Input: part model. Units: mm. Frame: model coordinates. A direction names the side the tool comes from. Round coordinates to 2 decimals unless told otherwise and drop trailing zeros. Answer as a JSON object with one key per item and string values.
```python
from build123d import *

# Parameters (mm, degrees)
SKETCH2_R           = 9.25
BOSS_EXTRUDE1_DEPTH = 4
SKETCH3_R           = 4.5
BOSS_EXTRUDE2_DEPTH = 1.2


with BuildPart() as part:
    # Sketch2 → Boss-Extrude1 (new, symmetric)
    with BuildSketch(Plane(origin=(0, 0, 0), x_dir=(1, 0, 0), z_dir=(0, 1, 0))):
        with BuildLine():
            Line((0.257214207, 22.945508076), (-9.742785793, 5.625))
            ThreePointArc((-9.742785793, 5.625), (-9.742785793, -5.625), (0, -11.25))
            Line((0, -11.25), (140, -11.25))
            ThreePointArc((140, -11.25), (145.625, -9.742785793), (149.742785793, -5.625))
            Line((149.742785793, -5.625), (159.742785793, 11.695508076))
            ThreePointArc((159.742785793, 11.695508076), (159.742785793, 22.945508076), (150, 28.570508076))
            Line((150, 28.570508076), (10, 28.570508076))
            ThreePointArc((10, 28.570508076), (4.375, 27.063293868), (0.257214207, 22.945508076))
        make_face()
        with Locations(Location((10, 17.320508076, 0), (0, 0, 270))):
            Circle(SKETCH2_R, mode=Mode.SUBTRACT)
        with Locations(Location((0, 0, 0), (0, 0, 270))):
            Circle(SKETCH2_R, mode=Mode.SUBTRACT)
        with Locations(Location((20, 0, 0), (0, 0, 270))):
            Circle(SKETCH2_R, mode=Mode.SUBTRACT)
        with Locations(Location((40, 0, 0), (0, 0, 270))):
            Circle(SKETCH2_R, mode=Mode.SUBTRACT)
        with Locations(Location((60, 0, 0), (0, 0, 270))):
            Circle(SKETCH2_R, mode=Mode.SUBTRACT)
        with Locations(Location((80, 0, 0), (0, 0, 270))):
            Circle(SKETCH2_R, mode=Mode.SUBTRACT)
        with Locations(Location((100, 0, 0), (0, 0, 270))):
            Circle(SKETCH2_R, mode=Mode.SUBTRACT)
        with Locations(Location((120, 0, 0), (0, 0, 270))):
            Circle(SKETCH2_R, mode=Mode.SUBTRACT)
        with Locations(Location((140, 0, 0), (0, 0, 270))):
            Circle(SKETCH2_R, mode=Mode.SUBTRACT)
        with Locations(Location((30, 17.320508076, 0), (0, 0, 270))):
            Circle(SKETCH2_R, mode=Mode.SUBTRACT)
        with Locations(Location((50, 17.320508076, 0), (0, 0, 270))):
            Circle(SKETCH2_R, mode=Mode.SUBTRACT)
        with Locations(Location((70, 17.320508076, 0), (0, 0, 270))):
            Circle(SKETCH2_R, mode=Mode.SUBTRACT)
        with Locations(Location((90, 17.320508076, 0), (0, 0, 270))):
            Circle(SKETCH2_R, mode=Mode.SUBTRACT)
        with Locations(Location((110, 17.320508076, 0), (0, 0, 270))):
            Circle(SKETCH2_R, mode=Mode.SUBTRACT)
        with Locations(Location((130, 17.320508076, 0), (0, 0, 270))):
            Circle(SKETCH2_R, mode=Mode.SUBTRACT)
        with Locations(Location((150, 17.320508076, 0), (0, 0, 270))):
            Circle(SKETCH2_R, mode=Mode.SUBTRACT)
    extrude(amount=BOSS_EXTRUDE1_DEPTH, both=True)

    # Sketch3 → Boss-Extrude2 (add)
    with BuildSketch(Plane(origin=(0, 4, 0), x_dir=(1, 0, 0), z_dir=(0, 1, 0))):
        with Locations(Location((10, 5.773502692, 0), (0, 0, 139.11591968))):
            Circle(SKETCH3_R)
        with Locations(Location((30, 5.773502692, 0), (0, 0, 40.88408032))):
            Circle(SKETCH3_R)
        with Locations(Location((50, 5.773502692, 0), (0, 0, 40.88408032))):
            Circle(SKETCH3_R)
        with Locations(Location((70, 5.773502692, 0), (0, 0, 40.88408032))):
            Circle(SKETCH3_R)
        with Locations(Location((90, 5.773502692, 0), (0, 0, 40.88408032))):
            Circle(SKETCH3_R)
        with Locations(Location((110, 5.773502692, 0), (0, 0, 40.88408032))):
            Circle(SKETCH3_R)
        with Locations(Location((130, 5.773502692, 0), (0, 0, 40.88408032))):
            Circle(SKETCH3_R)
        with BuildLine():
            Line((28.25, 28.570508076), (11.75, 28.570508076))
            add(Edge.make_bspline(
                [(11.75, 28.570508076), (11.75, 21.820508076), (20, 21.820508076), (28.25, 21.820508076), (28.25, 28.570508076)],
                knots=[3.141592654, 3.141592654, 3.141592654, 4.71238898, 4.71238898, 6.283185307, 6.283185307, 6.283185307], degree=2, weights=[1, 0.707106781, 1, 0.707106781, 1]))
        make_face()
        with BuildLine():
            Line((68.25, 28.570508076), (51.75, 28.570508076))
            add(Edge.make_bspline(
                [(51.75, 28.570508076), (51.75, 21.820508076), (60, 21.820508076), (68.25, 21.820508076), (68.25, 28.570508076)],
                knots=[3.141592654, 3.141592654, 3.141592654, 4.71238898, 4.71238898, 6.283185307, 6.283185307, 6.283185307], degree=2, weights=[1, 0.707106781, 1, 0.707106781, 1]))
        make_face()
        with BuildLine():
            Line((108.25, 28.570508076), (91.75, 28.570508076))
            add(Edge.make_bspline(
                [(91.75, 28.570508076), (91.75, 21.820508076), (100, 21.820508076), (108.25, 21.820508076), (108.25, 28.570508076)],
                knots=[3.141592654, 3.141592654, 3.141592654, 4.71238898, 4.71238898, 6.283185307, 6.283185307, 6.283185307], degree=2, weights=[1, 0.707106781, 1, 0.707106781, 1]))
        make_face()
        with BuildLine():
            Line((148.25, 28.570508076), (131.75, 28.570508076))
            add(Edge.make_bspline(
                [(131.75, 28.570508076), (131.75, 21.820508076), (140, 21.820508076), (148.25, 21.820508076), (148.25, 28.570508076)],
                knots=[3.141592654, 3.141592654, 3.141592654, 4.71238898, 4.71238898, 6.283185307, 6.283185307, 6.283185307], degree=2, weights=[1, 0.707106781, 1, 0.707106781, 1]))
        make_face()
        with BuildLine():
            Line((158.867785793, 10.179963619), (150.617785793, -4.109455543))
            add(Edge.make_bspline(
                [(158.867785793, 10.179963619), (153.022114317, 13.554963619), (148.897114317, 6.410254038), (144.772114317, -0.734455543), (150.617785793, -4.109455543)],
                knots=[0, 0, 0, 1.570796327, 1.570796327, 3.141592654, 3.141592654, 3.141592654], degree=2, weights=[1, 0.707106781, 1, 0.707106781, 1]))
        make_face()
    extrude(amount=BOSS_EXTRUDE2_DEPTH)


solid = part.part
```
1) Contact query for flat-ended pins moving along their axis: P1, Ø0.5, axis at x = 148, z = 0, coming from the -Y side; P2, Ø3, axis at y = -0.5, z = -24.5, coming from the +X side. Output: stop coordinate, or through.
Output:
{"P1": "stops at y = 4", "P2": "stops at x = 159.71"}
2) Section A-A, the plane y = 1.25. Count the separate pieces of the cut face and the enclosed holes in it, plus the area to 3 significant figures.
Output:
{"separate pieces": "1", "enclosed holes": "16", "area": "2,120 mm^2"}
3) Reachability of faces 1 (the face through (100.97, -0.06, -19.33)), 2 (the face through (-9.824, 0.056, 5.482)) from +Z, -Z, +X, -X, +Y, -Y: full face, straight path, thin tool, end or side. Return the list, or none.
Output:
{"face 1": "-Y", "face 2": "-X, +Y, -Y"}
4) Draft query along Z for faces 3 (the face through (145.553, 0.056, 9.784)), 4 (the face through (152, 5.2, -5)), 5 (the face through (120.97, -0.06, -19.33)), 6 (the face through (114.27, 4.59, -7.19)). Return one class per face: +Z half, -Z half, draft (parallel to the pull), parting line (faces both ways), or undercut.
Output:
{"face 3": "+Z half", "face 4": "draft", "face 5": "undercut", "face 6": "undercut"}
5) Ray query, probe 1 along Z at (x, y) = (10, -1.5); probe 2 along Z at (x, y) = (60, -1.5); probe 3 along Z at (x, y) = (77.5, 1.75). Return the intervals inside material, ascending.
Output:
{"probe 1": "z = -28.57 to -26.57, -8.07 to 11.25", "probe 2": "z = -28.57 to -9.25, 9.25 to 11.25", "probe 3": "z = -28.57 to -22.73, -11.91 to -8.91, 8.91 to 11.25"}
